Design review of the part built by this model. Coordinates are the model's own, in mm. A direction names the side the tool comes from. Coordinates: 2 decimals unless noted, no trailing zeros. Order: outer loops, then holes, each group sorted by start corner. A loop starts at its lowest first (then second) coordinate and runs counter-clockwise, first axis right, second up. Notation, with made-up numbers: M 45,-7.75 L 104,-7.75 A12 ccw 104,15.25 Z; hole C 84.25,36.5 d11. An arc over 180 degrees is marked long. Answer as a JSON object with one key per item and string values.
from build123d import *

# Parameters (mm, degrees)
EXTRUDE_1_DEPTH     = 5
SKETCH_2_W          = 16
SKETCH_2_H          = 6
EXTRUDE_2_DEPTH     = 1.5
SKETCH_3_R          = 1.35
CUT_EXTRUDE_1_DEPTH = 21.164572894
FILLET_1_R          = 1
FILLET_2_R          = 0.5


with BuildPart() as part:
    # 草图1 → 凸台-拉伸1 (new body)
    with BuildSketch(Plane.XY):
        Polygon((-12.6, 2.5), (-15.6, 2.5), (-15.6, -8.5), (15.6, -8.5), (15.6, 2.5), (12.6, 2.5), (12.6, -2.5), (-12.6, -2.5), align=None)
    extrude(amount=EXTRUDE_1_DEPTH)

    # 草图2 → 凸台-拉伸2 (add)
    with BuildSketch(Plane.XY.offset(5)):
        with Locations((0, -5.5)):
            Rectangle(SKETCH_2_W, SKETCH_2_H)
    extrude(amount=EXTRUDE_2_DEPTH)

    # 草图3 → 切除-拉伸1 (cut, through all)
    with BuildSketch(Plane.XZ.offset(8.5)):
        with Locations(Location((-6, 2.75, 0), (0, 0, 270))):
            Circle(SKETCH_3_R)
        with Locations((6, 2.75)):
            Circle(SKETCH_3_R)
    extrude(amount=-CUT_EXTRUDE_1_DEPTH, mode=Mode.SUBTRACT)

    # 圆角1
    fillet_1_edges = [part.edges().sort_by_distance(p)[0] for p in [
        (-8, -5.5, 5),
        (8, -5.5, 5),
    ]]
    fillet(fillet_1_edges, radius=FILLET_1_R)

    # 圆角2
    fillet_2_edges = [part.edges().sort_by_distance(p)[0] for p in [
        (15.6, -3, 0),
        (15.6, -3, 5),
        (8, -5.5, 6.5),
        (-8, -5.5, 6.5),
        (-15.6, -3, 5),
        (-15.6, -3, 0),
    ]]
    fillet(fillet_2_edges, radius=FILLET_2_R - 0.0001)  # a hair under: the kernel refuses the full size


solid = part.part
1) Add section A-A (z = 2.75). State the section outline as (x, y) points.
Taken from the geometry:
{"outline": "M -15.6,-8.5 L -7.35,-8.5 L -7.35,-2.5 L -12.6,-2.5 L -12.6,2.5 L -15.6,2.5 Z; M -4.65,-8.5 L 4.65,-8.5 L 4.65,-2.5 L -4.65,-2.5 Z; M 7.35,-8.5 L 15.6,-8.5 L 15.6,2.5 L 12.6,2.5 L 12.6,-2.5 L 7.35,-2.5 Z"}
2) To check wall thickness, follow L1, parallel to Z at x = 6, y = -5; L2, parallel to X at y = -1.75, z = 3.25; L3, parallel to X at y = -3.5, z = 2.25. State the ranges of each line that lie inside material, in increasing order.
Taken from the geometry:
{"L1": "z = 0 to 1.4, 4.1 to 6.5", "L2": "x = -15.6 to -12.6, 12.6 to 15.6", "L3": "x = -15.6 to -7.25, -4.75 to 4.75, 7.25 to 15.6"}
3) Tool access review of faces 1 (the flat face through (13, -4, 5)), 2 (the flat face through (-12.6, 0, 2)), 3 (the flat face through (-13, -4, 5)): name each direction out of +Z, -Z, +X, -X, +Y, -Y from which nothing blocks a thin tool from reaching the whole face with its end or side.
Taken from the geometry:
{"face 1": "+Z, +X, +Y, -Y", "face 2": "+Z, -Z, +Y", "face 3": "+Z, -X, +Y, -Y"}
4) Mouldability with a two-part tool opening along Z and no side actions: class faces 4 (the cylindrical face through (8.301, -5.458, 5.285)), 5 (the cylindrical face through (-5.594, -5.542, 1.462)), 6 (the cylindrical face through (6.62, -5.54, 1.55)), 7 (the flat face through (-14, 2.5, 2)) as released by +Z, released by -Z, zero draft, split by the parting line, or undercut.
Taken from the geometry:
{"face 4": "released by +Z", "face 5": "undercut", "face 6": "undercut", "face 7": "zero draft"}
5) Add section D-D (y = -1). State the section outline as (x, z) points, and give its area (3 significant figures).
Taken from the geometry:
{"outline": "M -15.6,0.5 A0.5 ccw -15.1,0 L -12.6,0 L -12.6,5 L -15.1,5 A0.5 ccw -15.6,4.5 Z; M 12.6,0 L 15.1,0 A0.5 ccw 15.6,0.5 L 15.6,4.5 A0.5 ccw 15.1,5 L 12.6,5 Z", "area": "29.8 mm2"}
6) Add section B-B (y = -7). Count the separate pieces of the cut face and the enclosed holes in it, and give its area (3 significant figures).
Taken from the geometry:
{"separate pieces": "1", "enclosed holes": "2", "area": "169 mm2"}
7) Add section C-C (x = -6). State the section outline as (y, z) points.
Taken from the geometry:
{"outline": "M -8.5,0 L -2.5,0 L -2.5,1.4 L -8.5,1.4 Z; M -8.5,4.1 L -2.5,4.1 L -2.5,6.5 L -8.5,6.5 Z"}
8) Insertion check: pin 1 Ø2.5 at (x, z) = (6, 2.75) entering from -Y; pin 2 Ø4 at (x, y) = (5.5, -1.5) entering from -Z; pin 3 Ø2 at (x, z) = (-5.5, 4) entering from +Y; pin 4 Ø1.8 at (x, y) = (-10.5, -2.5) entering from +Z. Each pin has a flat end and moves straight along its axis. Give the tip position at first contact, or say it passes through.
Taken from the geometry:
{"pin 1": "passes through", "pin 2": "stops at z = 0", "pin 3": "stops at y = -2.5", "pin 4": "stops at z = 5"}
